Geometry: final body of the model. Coordinates: model frame, mm. A direction names the side the tool comes from. Give positions to 0.01 mm unless a question says otherwise; leave off trailing zeros. Write each loop counter-clockwise with the first axis right and the second up, starting at its lowest first coordinate (ties: lowest second). Pieces come first, ordered by that corner, then holes. Notation, with made-up numbers: M -13.75,34.25 L 30.25,34.25 A4 ccw 30.25,39.25 Z; hole C -20.75,-24.75 d8. An arc over 180 degrees is marked long. Use a Markdown table: item, result. Add a question column.
1) Section C-C on y = 38. Return the cut outline in (x, z), then the cut area to 3 significant figures.
2) Line query: line 1 (Z direction, x = -10.75, y = 15); line 2 (X direction, y = 22, z = -11); line 3 (X direction, y = 15.5, z = 1.5). Output: solid intervals per line, ascending.
3) Section D-D on z = -17. Return the cut outline in (x, y), then the cut area to 3 significant figures.
4) Set-up query: faces 1 (the flat face through (-14.665, 24.983, -43.972)), 2 (the cylindrical face through (-9.48, 20.53, -5.09)), 3 (the flat face through (-8.58, 12.98, -43.97)). Return all of +Z, -Z, +X, -X, +Y, -Y with unobstructed straight access to the full face (end or side cutting, diameter ignored); none if empty.
5) Pin query (flat end, axial travel): pin 1 (8 mm diameter, centred on y = 24, z = -28, fed in from -X); pin 2 (6 mm diameter, centred on x = -21, z = -39.5, fed in from +Y); pin 3 (8 mm diameter, centred on y = 31.5, z = -3.5, fed in from +X); pin 4 (1.5 mm diameter, centred on x = -10.5, z = -23.5, fed in from -Y). Return the tip coordinate at first contact, or that it passes through.
6) Draft query along X for faces 4 (the cylindrical face through (-10.981, 4.003, 1.972)), 5 (the flat face through (-14.665, 24.983, 1.972)), 6 (the cylindrical face through (-17.225, 39.948, 2.028)), 7 (the flat face through (-14, 24, 4)). Return one class per face: +X half, -X half, draft (parallel to the pull), parting line (faces both ways), or undercut.
7) Section B-B on y = 43. Return the cut outline in (x, z).
8) Section A-A on x = -25. Return the cut outline in (y, z).
```python
from build123d import *

# Parameters (mm, degrees)
SKETCH1_R           = 2.5
BOSS_EXTRUDE1_DEPTH = 4
BOSS_EXTRUDE2_DEPTH = 50
SKETCH3_R           = 2
SKETCH3_R_2         = 1
CUT_EXTRUDE1_DEPTH  = 10
FILLET1_R           = 3


with BuildPart() as part:
    # Sketch1 → Boss-Extrude1 (new body)
    with BuildSketch(Plane.XY):
        with BuildLine():
            Line((-7.842362425, 10.716234493), (-17.397624454, 40.071064625))
            ThreePointArc((-17.397624454, 40.071064625), (-25.795005306, 45.357497095), (-18.956793202, 38.167140452))
            Line((-18.956793202, 38.167140452), (-18.754238897, 37.544871045))
            Line((-18.754238897, 37.544871045), (-10.63810017, 12.611188123))
            Line((-10.63810017, 12.611188123), (-10.256851829, 11.439950722))
            ThreePointArc((-10.256851829, 11.439950722), (-11.874437039, 1.653788416), (-7.842362425, 10.716234493))
        make_face()
        with Locations((-10.438845238, 6.44326398)):
            Circle(SKETCH1_R, mode=Mode.SUBTRACT)
        with Locations((-21.926625837, 42.189589224)):
            Circle(SKETCH1_R, mode=Mode.SUBTRACT)
    boss_extrude1 = extrude(amount=BOSS_EXTRUDE1_DEPTH)

    # Sketch2 → Boss-Extrude2 (add)
    with BuildSketch(Plane.XY.offset(4)):
        Polygon((-16.14843876, 36.233426921), (-9.957962302, 17.215593153), (-7.105287237, 18.144164622), (-13.295763695, 37.161998389), align=None)
    extrude(amount=-BOSS_EXTRUDE2_DEPTH)

    # Mirror1: Boss-Extrude1 across plane
    add(boss_extrude1.mirror(Plane.XY.offset(-21)))

    # Sketch3 → Cut-Extrude1 (cut)
    with BuildSketch(Plane(origin=(-3.936983875, -1.281523768, 0), x_dir=(0, 0, 1), z_dir=(-0.950891688393093, -0.30952382290371966, 0))):
        with Locations(Location((-5, 34.452391, 0), (0, 0, 270))):
            Circle(SKETCH3_R)
        with Locations(Location((-5, 24.452391, 0), (0, 0, 90))):
            Circle(SKETCH3_R)
        with Locations(Location((-37, 24.452391, 0), (0, 0, 270))):
            Circle(SKETCH3_R)
        with Locations(Location((-37, 34.452391, 0), (0, 0, 90))):
            Circle(SKETCH3_R)
        with Locations(Location((-21, 29.452391, 0), (0, 0, 270))):
            Circle(SKETCH3_R_2)
    extrude(amount=-CUT_EXTRUDE1_DEPTH, mode=Mode.SUBTRACT)

    # Fillet1
    fillet1_edges = [part.edges().sort_by_distance(p)[0] for p in [
        (-9.957962302, 17.215593153, 2),
        (-9.957962302, 17.215593153, -44),
        (-16.14843876, 36.233426921, -44),
        (-16.14843876, 36.233426921, 2),
        (-10.256851829, 11.439950722, 2),
        (-7.842362425, 10.716234493, 2),
        (-7.842362425, 10.716234493, -44),
        (-10.256851829, 11.439950722, -44),
        (-17.397624454, 40.071064625, -44),
        (-18.956793202, 38.167140452, -44),
        (-17.397624454, 40.071064625, 2),
        (-18.956793202, 38.167140452, 2),
    ]]
    fillet(fillet1_edges, radius=FILLET1_R - 0.0001)  # a hair under: the kernel refuses the full size


solid = part.part
```
Found:
| question | item | result |
|---|---|---|
| 1 | outline | M -24.66,-46 L -16.45,-46 L -16.45,-42 L -24.66,-42 Z; M -24.66,0 L -16.45,0 L -16.45,4 L -24.66,4 Z |
| 1 | area | 65.7 mm² |
| 2 | line 1 | -46 to -42, 0 to 4 |
| 2 | line 2 | -11.52 to -8.36 |
| 2 | line 3 | -11.58 to -9.17 |
| 3 | outline | M -16.15,36.23 L -9.96,17.22 L -7.11,18.14 L -13.3,37.16 Z |
| 3 | area | 60.0 mm² |
| 4 | face 1 | +Z, -Z, -X |
| 4 | face 2 | none |
| 4 | face 3 | +Z, -Z, +X |
| 5 | pin 1 | x = -13.47 |
| 5 | pin 2 | y = 47.19 |
| 5 | pin 3 | x = -10.15 |
| 5 | pin 4 | y = 17.22 |
| 6 | face 4 | undercut |
| 6 | face 5 | -X half |
| 6 | face 6 | +X half |
| 6 | face 7 | draft |
| 7 | outline | M -26.86,-46 L -24.29,-46 L -24.29,-42 L -26.86,-42 Z; M -26.86,0 L -24.29,0 L -24.29,4 L -26.86,4 Z; M -19.56,-46 L -16.99,-46 L -16.99,-42 L -19.56,-42 Z; M -19.56,0 L -16.99,0 L -16.99,4 L -19.56,4 Z |
| 8 | outline | M 38.25,-46 L 46.13,-46 L 46.13,-42 L 38.25,-42 Z; M 38.25,0 L 46.13,0 L 46.13,4 L 38.25,4 Z |
